```python
from build123d import *

# Parameters (mm, degrees)
SKETCH2_R           = 2
BOSS_EXTRUDE1_DEPTH = 8
CHAMFER1_SIZE       = 0.5
CUT_EXTRUDE1_DEPTH  = 2.3
SKETCH8_R           = 1.782050808
CUT_EXTRUDE2_DEPTH  = 1
CUT_EXTRUDE2_TAPER  = 45


with BuildPart() as part:
    # Sketch2 → Boss-Extrude1 (new body)
    with BuildSketch(Plane(origin=(0, 0, 0), x_dir=(0, 0, -1), z_dir=(1, 0, 0))):
        Circle(SKETCH2_R)
    extrude(amount=-BOSS_EXTRUDE1_DEPTH)

    # Chamfer1
    chamfer1_edges = [part.edges().sort_by_distance(p)[0] for p in [
        (0, 0, 2),
    ]]
    chamfer(chamfer1_edges, length=CHAMFER1_SIZE)

    # Sketch6 → Revolve1 (revolve)
    with BuildSketch(Plane.XY):
        with BuildLine():
            Line((-9.5, 0), (-9.5, 4.161437828))
            ThreePointArc((-9.5, 4.161437828), (-8.75, 4.5), (-8, 4.161437828))
            Line((-8, 4.161437828), (-8, 0))
            Line((-8, 0), (-9.5, 0))
        make_face()
    revolve(axis=Axis((-8, 0, 0), (-1, 0, 0)))

    # Sketch7 → Cut-Extrude1 (cut)
    with BuildSketch(Plane.ZY.offset(9.5)):
        Polygon((0, 1.732050808), (-1.5, 0.866025404), (-1.5, -0.866025404), (0, -1.732050808), (1.5, -0.866025404), (1.5, 0.866025404), align=None)
    extrude(amount=-CUT_EXTRUDE1_DEPTH, mode=Mode.SUBTRACT)

    # Sketch8 → Cut-Extrude2 (cut)
    with BuildSketch(Plane.ZY.offset(9.5)):
        Circle(SKETCH8_R)
    extrude(amount=-CUT_EXTRUDE2_DEPTH, taper=CUT_EXTRUDE2_TAPER, mode=Mode.SUBTRACT)


solid = part.part
```
Geometry: final body of the model. Coordinates: model frame, mm. A direction names the side the tool comes from. Coordinates: 2 decimals unless noted, no trailing zeros. Order: outer loops, then holes, each group sorted by start corner. A loop starts at its lowest first (then second) coordinate and runs counter-clockwise, first axis right, second up. Notation, with made-up numbers: M -9.75,-6 L 22.25,-6 A18 ccw 22.25,-2 Z; hole C 48.5,30.25 d8. An arc over 180 degrees is marked long. Answer in a Markdown table with one row per item. Add a question column.
Q1. Contact query for flat-ended pins moving along their axis: P1, Ø1.5, axis at x = -2, z = -1, coming from the -Y side; P2, Ø2, axis at x = -5, y = 0.5, coming from the -Z side; P3, Ø5, axis at x = -2.5, z = 3, coming from the -Y side. Output: stop coordinate, or through.
Q2. Section query A-A on x = -3. Return the cut outline in (y, z), and give its area (3 significant figures).
Q3. Mould query, pull axis Z, two halves, no side actions, for faces 4 (the flat face through (-9.5, -2, 0)), 5 (the flat face through (-8, 0, 1.5)), 6 (the cylindrical face through (-4, -2, 0)). Classes: released by +Z, released by -Z, zero draft, split by the parting line, or undercut.
Q4. Reachability of faces 1 (the flat face through (-7.2, 0, 0)), 2 (the flat face through (0, 0, 0)), 3 (the flat face through (-8, 2, -1)) from +Z, -Z, +X, -X, +Y, -Y: full face, straight path, thin tool, end or side. Return the list, or none.
Q5. Line query: L1, parallel to X at y = -3, z = -2.25; L2, parallel to Y at x = -2.5, z = 0; L3, parallel to Z at x = -4.5, y = -1. Output: solid intervals per line, ascending.
Completed:
| question | item | result |
|---|---|---|
| 1 | P1 | stops at y = -1.98 |
| 1 | P2 | stops at z = -2 |
| 1 | P3 | stops at y = -1.94 |
| 2 | outline | C 0,0 d4 |
| 2 | area | 12.6 mm2 |
| 3 | face 4 | zero draft |
| 3 | face 5 | undercut |
| 3 | face 6 | split by the parting line |
| 4 | face 1 | -X |
| 4 | face 2 | +Z, -Z, +X, +Y, -Y |
| 4 | face 3 | +X |
| 5 | L1 | x = -9.5 to -8 |
| 5 | L2 | y = -2 to 2 |
| 5 | L3 | z = -1.73 to 1.73 |
